Design review of the part built by this model. Coordinates are the model's own, in mm. A direction names the side the tool comes from. Round coordinates to 2 decimals unless told otherwise and drop trailing zeros. Loops run counter-clockwise (first coordinate to the right, second up) from the corner with the lowest first, then second, coordinate; pieces in that order, holes last. Notation, with made-up numbers: M -1,43.5 L 8,43.5 A22 ccw 8,63.5 Z; hole C -19.5,21.25 d4. An arc over 180 degrees is marked long. One line per item, written item: value. Start each with the question number.
Item 1: We need section A-A (z = -190.5). Write out the cut boundary in (x, y), then the cut area to 3 significant figures.
Item 2: Clearance check with flat-ended pins moving along their axes: pin 1 (14.5 mm diameter, centred on x = 58.5, z = -101.5, fed in from +Y); pin 2 (1.5 mm diameter, centred on x = 37, z = -97.5, fed in from -Y); pin 3 (3 mm diameter, centred on x = 68, y = 7, fed in from +Z); pin 4 (2.5 mm diameter, centred on x = -67.5, y = -88, fed in from -Z). State where each tip first meets the part, or that it passes through.
Item 3: We need section C-C (x = -73). Write out the cut boundary in (y, z) (3 decimals).
Item 4: For faces 5 (the flat face through (-1, -88.9, -119)), 6 (the flat face through (33.874, -81, -119)), 7 (the flat face through (-33.874, -81, -119)), list the 3-axis set-ups (+Z, -Z, +X, -X, +Y, -Y) from which the entire face can be reached by the end or side of a thin tool; tool diameter is ignored.
Item 5: For line 1 along Z through (x, y) = (64, -64) (3 decimals); line 2 along X through (y, z) = (-82, -144); line 3 along X through (y, z) = (-18.5, -104.5), list the stretches that pass through material, from the lowest coordinate up.
Item 6: Mouldability with a two-part tool opening along Z and no side actions: class faces 1 (the flat face through (-1, 1, 0)), 2 (the flat face through (1, 1, -285.75)), 3 (the flat face through (0, -85, -203.2)), 4 (the flat face through (58, -85.979, -119)) as released by +Z, released by -Z, zero draft, split by the parting line, or undercut.
Item 7: We need section D-D (z = -47). Write out the cut boundary in (x, y), then the cut area to 3 significant figures.
Item 8: We need section B-B (y = 0). Write out the cut boundary in (x, z) (3 decimals).
from build123d import *

# Parameters (mm, degrees)
SKETCH1_R           = 82.4992
BOSS_EXTRUDE1_DEPTH = 285.75
SKETCH2_R           = 95.25
BOSS_EXTRUDE2_DEPTH = 47.625
SKETCH3_W           = 164.9984
SKETCH3_H           = 2.921
BOSS_EXTRUDE3_DEPTH = 165.1
CUT_EXTRUDE1_REACH  = 353.525


with BuildPart() as part:
    # Sketch1 → Boss-Extrude1 (new body)
    with BuildSketch(Plane.XY):
        Circle(SKETCH1_R)
    extrude(amount=-BOSS_EXTRUDE1_DEPTH)

    # Sketch2 → Boss-Extrude2 (add)
    with BuildSketch(Plane(origin=(0, 0, -285.75), x_dir=(-1, 0, 0), z_dir=(0, 0, -1))):
        Circle(SKETCH2_R)
    extrude(amount=-BOSS_EXTRUDE2_DEPTH)

    # Sketch3 → Boss-Extrude3 (add)
    with BuildSketch(Plane.XY.offset(-38.1)):
        with BuildLine():
            Line((-33.873610408, -85.979), (33.873610408, -85.979))
            Line((33.873610408, -85.979), (33.873610408, -75.22430803))
            ThreePointArc((33.873610408, -75.22430803), (0, -82.4992), (-33.873610408, -75.22430803))
            Line((-33.873610408, -75.22430803), (-33.873610408, -85.979))
        make_face()
        with Locations((0, -87.4395)):
            Rectangle(SKETCH3_W, SKETCH3_H)
    extrude(amount=-BOSS_EXTRUDE3_DEPTH)

    # Sketch4 → Cut-Extrude1 (cut, up to next)
    with BuildSketch(Plane(origin=(0, -85.979, 0), x_dir=(1, 0, 0), z_dir=(0, 1, 0)), mode=Mode.PRIVATE) as cut_extrude1_sk1:
        with BuildLine():
            Line((-76.1492, 67.691), (-50.7492, 67.691))
            ThreePointArc((-50.7492, 67.691), (-46.5582, 63.5), (-50.7492, 59.309))
            Line((-50.7492, 59.309), (-76.1492, 59.309))
            ThreePointArc((-76.1492, 59.309), (-80.3402, 63.5), (-76.1492, 67.691))
        make_face()
    cut_extrude1_tool1 = extrude(cut_extrude1_sk1.sketch, amount=-CUT_EXTRUDE1_REACH, mode=Mode.PRIVATE) & part.part
    # Sketch4 → Cut-Extrude1 (cut, up to next)
    with BuildSketch(Plane(origin=(0, -85.979, 0), x_dir=(1, 0, 0), z_dir=(0, 1, 0)), mode=Mode.PRIVATE) as cut_extrude1_sk2:
        with BuildLine():
            Line((-50.7492, 186.309), (-76.1492, 186.309))
            ThreePointArc((-76.1492, 186.309), (-80.3402, 190.5), (-76.1492, 194.691))
            Line((-76.1492, 194.691), (-50.7492, 194.691))
            ThreePointArc((-50.7492, 194.691), (-46.5582, 190.5), (-50.7492, 186.309))
        make_face()
    cut_extrude1_tool2 = extrude(cut_extrude1_sk2.sketch, amount=-CUT_EXTRUDE1_REACH, mode=Mode.PRIVATE) & part.part
    cut_extrude1_1 = cut_extrude1_tool1.solids().sort_by_distance((-63.4492, -85.979, -63.5))[0]
    add(cut_extrude1_1, mode=Mode.SUBTRACT)
    cut_extrude1_2 = cut_extrude1_tool2.solids().sort_by_distance((-63.4492, -85.979, -190.5))[0]
    add(cut_extrude1_2, mode=Mode.SUBTRACT)
    cut_extrude1 = cut_extrude1_1 + cut_extrude1_2  # Cut-Extrude1 as one shape, for the pattern or mirror that repeats it

    # Mirror1: Cut-Extrude1 across plane
    add(cut_extrude1.mirror(Plane(origin=(0, 0, 0), x_dir=(0, 0, 1), z_dir=(1, 0, 0))), mode=Mode.SUBTRACT)


solid = part.part
A:
1. outline: M -82.5,-88.9 L -80.34,-88.9 L -80.34,-85.98 L -82.5,-85.98 Z; M -46.56,-88.9 L 46.56,-88.9 L 46.56,-85.98 L 33.87,-85.98 L 33.87,-75.22 A82.5 ccw long -33.87,-75.22 L -33.87,-85.98 L -46.56,-85.98 Z; M 80.34,-88.9 L 82.5,-88.9 L 82.5,-85.98 L 80.34,-85.98 Z
1. area: 22,100 mm2
2. pin 1: y = 64.65
2. pin 2: y = -88.9
2. pin 3: z = 0
2. pin 4: z = -203.2
3. outline: M -88.9,-203.2 L -85.979,-203.2 L -85.979,-194.691 L -88.9,-194.691 Z; M -88.9,-186.309 L -85.979,-186.309 L -85.979,-67.691 L -88.9,-67.691 Z; M -88.9,-59.309 L -85.979,-59.309 L -85.979,-38.1 L -88.9,-38.1 Z; M -61.185,-285.75 L 61.185,-285.75 L 61.185,-238.125 L 38.433,-238.125 L 38.433,0 L -38.433,0 L -38.433,-238.125 L -61.185,-238.125 Z
4. face 5: +Z, +X, -X, -Y
4. face 6: +Z, +X
4. face 7: +Z, -X
5. line 1: -285.75 to -238.125
5. line 2: -33.87 to 33.87
5. line 3: -80.4 to 80.4
6. face 1: released by +Z
6. face 2: released by -Z
6. face 3: undercut
6. face 4: zero draft
7. outline: M -82.5,-88.9 L 82.5,-88.9 L 82.5,-85.98 L 33.87,-85.98 L 33.87,-75.22 A82.5 ccw long -33.87,-75.22 L -33.87,-85.98 L -82.5,-85.98 Z
7. area: 22,300 mm2
8. outline: M -95.25,-285.75 L 95.25,-285.75 L 95.25,-238.125 L 82.499,-238.125 L 82.499,0 L -82.499,0 L -82.499,-238.125 L -95.25,-238.125 Z
